Verification items for the finished model (mm, model axes). A direction names the side the tool comes from. Round coordinates to 2 decimals unless told otherwise and drop trailing zeros. Write each loop counter-clockwise with the first axis right and the second up, starting at its lowest first coordinate (ties: lowest second). Pieces come first, ordered by that corner, then holes. Notation, with made-up numbers: (-20, 59) -> (2, 59) arc R22 ccw to (2, 85) -> close; hole circle Ø2 at (69, 30.25). An arc over 180 degrees is marked (long way). Use CSV: the item, a comma, the result in double quotes.
```python
from build123d import *

# Parameters (mm, degrees)
MODEL_R             = 2
MODEL_R_2           = 2.5
BOSS_EXTRUDE1_DEPTH = 3


with BuildPart() as part:
    # Model → Boss-Extrude1 (new body)
    with BuildSketch(Plane.XY):
        with BuildLine():
            Line((-2, 30), (-48, 30))
            ThreePointArc((-48, 30), (-49.414213562, 29.414213562), (-50, 28))
            Line((-50, 28), (-50, 2))
            ThreePointArc((-50, 2), (-49.414213562, 0.585786438), (-48, 0))
            Line((-48, 0), (-2, 0))
            ThreePointArc((-2, 0), (-0.585786438, 0.585786438), (0, 2))
            Line((0, 2), (0, 28))
            ThreePointArc((0, 28), (-0.585786438, 29.414213562), (-2, 30))
        make_face()
        with Locations((-25, 15)):
            Circle(MODEL_R, mode=Mode.SUBTRACT)
        with Locations((-37.81005651, 8)):
            Circle(MODEL_R, mode=Mode.SUBTRACT)
        with Locations((-12.5, 8)):
            Circle(MODEL_R, mode=Mode.SUBTRACT)
        with Locations((-37.81005651, 22)):
            Circle(MODEL_R, mode=Mode.SUBTRACT)
        with Locations((-12.5, 22)):
            Circle(MODEL_R, mode=Mode.SUBTRACT)
        with Locations((-25, 8)):
            Circle(MODEL_R, mode=Mode.SUBTRACT)
        with Locations((-25, 22)):
            Circle(MODEL_R, mode=Mode.SUBTRACT)
        with Locations((-9, 15)):
            Circle(MODEL_R_2, mode=Mode.SUBTRACT)
        with Locations((-41, 15)):
            Circle(MODEL_R_2, mode=Mode.SUBTRACT)
        with BuildLine():
            Line((-21.884771632, 1), (-27.884771632, 1))
            ThreePointArc((-27.884771632, 1), (-28.884771632, 2), (-27.884771632, 3))
            Line((-27.884771632, 3), (-21.884771632, 3))
            ThreePointArc((-21.884771632, 3), (-20.884771632, 2), (-21.884771632, 1))
        make_face(mode=Mode.SUBTRACT)
        with BuildLine():
            Line((-28, 28.999828109), (-22, 28.999828109))
            ThreePointArc((-22, 28.999828109), (-21, 27.999828109), (-22, 26.999828109))
            Line((-22, 26.999828109), (-28, 26.999828109))
            ThreePointArc((-28, 26.999828109), (-29, 27.999828109), (-28, 28.999828109))
        make_face(mode=Mode.SUBTRACT)
    extrude(amount=BOSS_EXTRUDE1_DEPTH)


solid = part.part
```
Q1. Section check C-C (z = 1.1). State how many separate pieces and enclosed holes the cut face has, plus the area to 3 significant figures.
Filled in:
separate pieces,"1"
enclosed holes,"11"
area,"1,340 mm²"
Q2. Go/stop test with a flat-tipped pin: P1, Ø4.5, axis at x = -9, y = 15, coming from the -Z side. Record where the tip stops, or that it passes through.
Filled in:
P1,"through"
Q3. Section check D-D (y = 8). Record the cut outline in (x, z).
Filled in:
outline,"(-50, 0) -> (-39.81, 0) -> (-39.81, 3) -> (-50, 3) -> close; (-35.81, 0) -> (-27, 0) -> (-27, 3) -> (-35.81, 3) -> close; (-23, 0) -> (-14.5, 0) -> (-14.5, 3) -> (-23, 3) -> close; (-10.5, 0) -> (0, 0) -> (0, 3) -> (-10.5, 3) -> close"
Q4. Section check B-B (y = 15). Record the cut outline in (x, z), plus the area to 3 significant figures.
Filled in:
outline,"(-50, 0) -> (-43.5, 0) -> (-43.5, 3) -> (-50, 3) -> close; (-38.5, 0) -> (-27, 0) -> (-27, 3) -> (-38.5, 3) -> close; (-23, 0) -> (-11.5, 0) -> (-11.5, 3) -> (-23, 3) -> close; (-6.5, 0) -> (0, 0) -> (0, 3) -> (-6.5, 3) -> close"
area,"108 mm²"
Q5. Material ranges on L1, parallel to Y at x = -25, z = 1.6; L2, parallel to Y at x = -12.5, z = 0.9; L3, parallel to Y at x = -9, z = 1.8, recorded low to high.
Filled in:
L1,"0 to 1, 3 to 6, 10 to 13, 17 to 20, 24 to 27, 29 to 30"
L2,"0 to 6, 10 to 20, 24 to 30"
L3,"0 to 12.5, 17.5 to 30"
Q6. Section check A-A (x = -9). Record the cut outline in (y, z), plus the area to 3 significant figures.
Filled in:
outline,"(0, 0) -> (12.5, 0) -> (12.5, 3) -> (0, 3) -> close; (17.5, 0) -> (30, 0) -> (30, 3) -> (17.5, 3) -> close"
area,"75.0 mm²"
Q7. Mould release check, pull along X, two halves, no side actions. Record for faces 1 (the cylindrical face through (-38.69, 14.04, 1.48)), 2 (the flat face through (-25, 12, 3)), 3 (the flat face through (-50, 15, 1)), 4 (the cylindrical face through (-39.81, 22.09, 1.48)): released by +X, released by -X, zero draft, split by the parting line, or undercut.
Filled in:
face 1,"undercut"
face 2,"zero draft"
face 3,"released by -X"
face 4,"undercut"
Q8. Access from +Z, -Z, +X, -X, +Y, -Y to the whole of each face (thin tool, end or side, straight path). Record for faces 5 (the flat face through (0, 15, 1)), 6 (the flat face through (-25, 1, 1)).
Filled in:
face 5,"+Z, -Z, +X, +Y, -Y"
face 6,"+Z, -Z"
